from build123d import *

# Parameters (mm, degrees)
SKETCH_1_R          = 3
SKETCH_1_R_2        = 1.5
EXTRUDE_1_DEPTH     = 5
EXTRUDE_2_DEPTH     = 5
SKETCH_4_R          = 1.5
CUT_EXTRUDE_1_DEPTH = 144.265487819
EXTRUDE_START       = -5
EXTRUDE_3_DEPTH     = 5
CUT_EXTRUDE_2_DEPTH = 144.265487819
SKETCH_7_R          = 1.6
CUT_EXTRUDE_3_DEPTH = 144.265487819


with BuildPart() as part:
    # 草图1 → 凸台-拉伸1 (new body)
    with BuildSketch(Plane.XY):
        with BuildLine():
            Line((-3.933140204, 6.966376973), (90, 60))
            Line((90, 60), (130, 60))
            Line((130, 60), (130, 30))
            Line((130, 30), (92, 30))
            Line((92, 30), (3.100465808, -7.374761811))
            ThreePointArc((3.100465808, -7.374761811), (-7.182645896, -3.522725923), (-3.933140204, 6.966376973))
        make_face()
        Circle(SKETCH_1_R, mode=Mode.SUBTRACT)
        with Locations((95, 55)):
            Circle(SKETCH_1_R_2, mode=Mode.SUBTRACT)
        with Locations((125, 55)):
            Circle(SKETCH_1_R_2, mode=Mode.SUBTRACT)
        with Locations((125, 35)):
            Circle(SKETCH_1_R_2, mode=Mode.SUBTRACT)
        with Locations((95, 35)):
            Circle(SKETCH_1_R_2, mode=Mode.SUBTRACT)
    extrude(amount=EXTRUDE_1_DEPTH)

    # 草图3 → 凸台-拉伸2 (add)
    with BuildSketch(Plane.XY.offset(5)):
        Polygon((81.144001216, 55), (20, 55), (20, 20.478766027), align=None)
    extrude(amount=-EXTRUDE_2_DEPTH)

    # 草图4 → 切除-拉伸1 (cut, through all)
    with BuildSketch(Plane.XY.offset(5)):
        with Locations((25, 52)):
            Circle(SKETCH_4_R)
        with Locations((45, 52)):
            Circle(SKETCH_4_R)
    extrude(amount=-CUT_EXTRUDE_1_DEPTH, mode=Mode.SUBTRACT)

    # 草图6 → 凸台-拉伸3 (add)
    with BuildSketch(Plane.XY.offset(5).offset(EXTRUDE_START)):
        with BuildLine():
            Line((-7.074049095, 3.736017853), (20, 55))
            Line((20, 55), (20, 20.478766027))
            Line((20, 20.478766027), (-3.933140204, 6.966376973))
            ThreePointArc((-3.933140204, 6.966376973), (-5.735709118, 5.576884517), (-7.074049095, 3.736017853))
        make_face()
    extrude(amount=EXTRUDE_3_DEPTH)

    # 草图5 → 切除-拉伸2 (cut, through all)
    with BuildSketch(Plane.XY.offset(5)):
        with BuildLine():
            Line((105, 52), (115, 52))
            ThreePointArc((115, 52), (122, 45), (115, 38))
            Line((115, 38), (105, 38))
            ThreePointArc((105, 38), (98, 45), (105, 52))
        make_face()
        with BuildLine():
            Line((25.605401824, 44.200503347), (15.042800964, 24.200503347))
            ThreePointArc((15.042800964, 24.200503347), (15.293877797, 22.454192152), (17.032531201, 22.154647985))
            Line((17.032531201, 22.154647985), (57.595132061, 42.154647985))
            ThreePointArc((57.595132061, 42.154647985), (58.392612512, 43.840567158), (56.93178603, 45))
            Line((56.93178603, 45), (26.93178603, 45))
            ThreePointArc((26.93178603, 45), (26.157433081, 44.784670195), (25.605401824, 44.200503347))
        make_face()
    extrude(amount=-CUT_EXTRUDE_2_DEPTH, mode=Mode.SUBTRACT)

    # 草图7 → 切除-拉伸3 (cut, through all)
    with BuildSketch(Plane.XY.offset(5)):
        with Locations((10, 18)):
            Circle(SKETCH_7_R)
        with Locations((30, 18)):
            Circle(SKETCH_7_R)
    extrude(amount=-CUT_EXTRUDE_3_DEPTH, mode=Mode.SUBTRACT)


solid = part.part
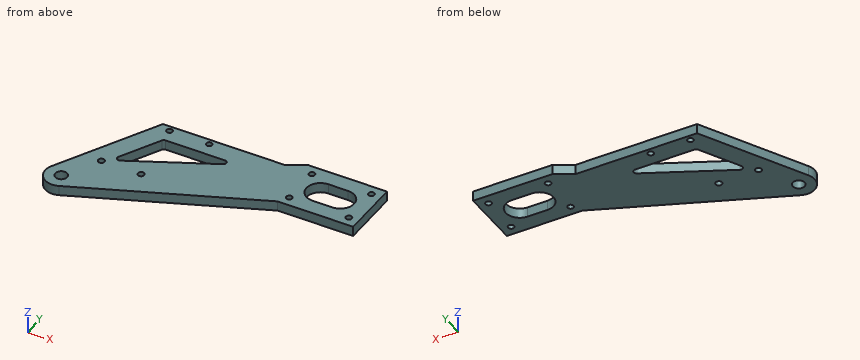
Check sheet for the modelled part. Datum: model origin and axes. Units: mm. Give positions to 0.01 mm unless a question says otherwise; leave off trailing zeros. Write each loop counter-clockwise with the first axis right and the second up, starting at its lowest first coordinate (ties: lowest second). Pieces come first, ordered by that corner, then holes. Notation, with made-up numbers: (9.25, 31) -> (18.25, 31) arc R34 ccw to (18.25, 67) -> close; hole circle Ø10 at (5.25, -34). An arc over 180 degrees is marked (long way). Use one line per item in the form item = value. Start each with the question number.
1. Go/stop test with flat-tipped pins: P1, Ø1.5, axis at x = 111, z = 2, coming from the -Y side; P2, Ø2.5, axis at x = 38.5, z = 3, coming from the +Y side. Record where each tip stops, or that it passes through.
2. Section check A-A (x = 125). Record the cut outline in (y, z), and give its area (3 significant figures).
3. Thickness scan on line 1 along Y through (x, z) = (125, 2.75); line 2 along Y through (x, z) = (112, 2.15); line 3 along Y through (x, z) = (29.5, 4.05). Record the ranges inside material, lowest first. Write a range as from..to.
4. Section check C-C (x = 10). Record the cut outline in (y, z), and give its area (3 significant figures).
5. Section check D-D (y = 0). Record the cut outline in (x, z), and give its area (3 significant figures).
6. Section check B-B (z = 1.9). Count the separate pieces of the cut face and the enclosed holes in it, and give its area (3 significant figures).
Conclusion:
q1.P1 = 30
q1.P2 = 55
q2.outline = (30, 0) -> (33.5, 0) -> (33.5, 5) -> (30, 5) -> close; (36.5, 0) -> (53.5, 0) -> (53.5, 5) -> (36.5, 5) -> close; (56.5, 0) -> (60, 0) -> (60, 5) -> (56.5, 5) -> close
q2.area = 120 mm²
q3.line_1 = 30..33.5, 36.5..53.5, 56.5..60
q3.line_2 = 30..38, 52..60
q3.line_3 = 3.72..16.48, 19.52..28.3, 45..55
q4.outline = (-4.47, 0) -> (16.4, 0) -> (16.4, 5) -> (-4.47, 5) -> close; (19.6, 0) -> (36.07, 0) -> (36.07, 5) -> (19.6, 5) -> close
q4.area = 187 mm²
q5.outline = (-8, 0) -> (-3, 0) -> (-3, 5) -> (-8, 5) -> close; (3, 0) -> (20.64, 0) -> (20.64, 5) -> (3, 5) -> close
q5.area = 113 mm²
q6.separate_pieces = 1
q6.enclosed_holes = 11
q6.area = 4,160 mm²
